```python
from build123d import *

# Parameters (mm, degrees)
SKETCH1_R           = 12.7
BOSS_EXTRUDE1_DEPTH = 58.7248
CHAMFER3_SIZE       = 6.35
CHAMFER3_SIZE2      = 23.698522628
CHAMFER4_SIZE       = 6.35
CHAMFER4_SIZE2      = 23.698522628
CUT_EXTRUDE1_DEPTH  = 58.7248
SKETCH3_R           = 1.5875
CUT_EXTRUDE2_DEPTH  = 62.409951433


with BuildPart() as part:
    # Sketch1 → Boss-Extrude1 (new body)
    with BuildSketch(Plane.XY):
        Circle(SKETCH1_R)
    extrude(amount=-BOSS_EXTRUDE1_DEPTH)

    # Chamfer3
    chamfer3_edges = [part.edges().sort_by_distance(p)[0] for p in [
        (-12.7, 0, -58.7248),
    ]]
    chamfer3_side = [part.faces().sort_by_distance(p)[0] for p in [
        (0, 0, -58.7248),
    ]]
    chamfer(chamfer3_edges, length=CHAMFER3_SIZE, length2=CHAMFER3_SIZE2, reference=chamfer3_side[0])

    # Chamfer4
    chamfer4_edges = [part.edges().sort_by_distance(p)[0] for p in [
        (-12.7, 0, 0),
    ]]
    chamfer4_side = [part.faces().sort_by_distance(p)[0] for p in [
        (0, 0, 0),
    ]]
    chamfer(chamfer4_edges, length=CHAMFER4_SIZE, length2=CHAMFER4_SIZE2, reference=chamfer4_side[0])

    # Sketch2 → Cut-Extrude1 (cut)
    with BuildSketch(Plane(origin=(0, 0, 0), x_dir=(1, 0, 0), z_dir=(0, 1, 0))):
        Polygon((-6.35, 0), (-12.7, 23.698522628), (-12.7, 35.026277372), (-6.35, 58.7248), (6.35, 58.7248), (12.7, 35.026277372), (12.7, 23.698522628), (6.35, 0), align=None)
    extrude(amount=-CUT_EXTRUDE1_DEPTH, mode=Mode.SUBTRACT)

    # Sketch3 → Cut-Extrude2 (cut, through all)
    with BuildSketch(Plane(origin=(0, 0, 0), x_dir=(1, 0, 0), z_dir=(0, 1, 0))):
        with Locations(Location((-10.16, 35.026277372, 0), (0, 0, 179.999999983))):
            Circle(SKETCH3_R)
        with Locations(Location((10.16, 35.026277372, 0), (0, 0, 90))):
            Circle(SKETCH3_R)
        with Locations((10.16, 23.698522628)):
            Circle(SKETCH3_R)
        with Locations(Location((-10.16, 23.698522628, 0), (0, 0, 90))):
            Circle(SKETCH3_R)
    extrude(amount=CUT_EXTRUDE2_DEPTH, mode=Mode.SUBTRACT)


solid = part.part
```
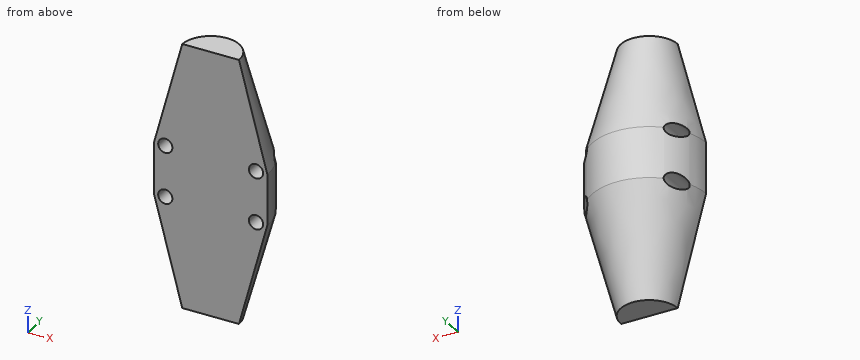
Here's how the part is built. I have some questions about the finished solid (model axes, mm). Coordinates: 2 decimals unless noted, no trailing zeros. Order: outer loops, then holes, each group sorted by start corner. A loop starts at its lowest first (then second) coordinate and runs counter-clockwise, first axis right, second up. Notation, with made-up numbers: M -29.75,-36.75 L 13.25,-36.75 A26 ccw 13.25,-3.75 Z; hole C 18,-3 d10. An arc over 180 degrees is marked long. Answer as a JSON object with one key per item and string values. Group by question number.
(1) Suppose I cut it at A-A, the plane x = 0. Please give me the cut outline in (y, z), then the cut area to 3 significant figures.
(2) Suppose I cut it at B-B, the plane y = 4. State how many separate pieces and enclosed holes the cut face has, then the cut area to 3 significant figures.
(3) For pin 1 (3 mm diameter, centred on x = -9, z = -27.5, fed in from -Y); pin 2 (2 mm diameter, centred on y = 11, z = -41.5, fed in from +X); pin 3 (1.5 mm diameter, centred on y = 8.5, z = -39.5, fed in from +X); pin 4 (3 mm diameter, centred on y = 2.5, z = -42.5, fed in from -X), each with a flat end and sliding along its axis, tell me the tip position at first contact or that it passes through.
(4) I need wall thicknesses on probe 1 along X at (y, z) = (1.5, -36); probe 2 along Y at (x, z) = (-4.25, -10); probe 3 along Y at (x, z) = (8.75, -31.5). Which ranges of each line are inside material? Lowest first, please.
(5) Suppose I cut it at D-D, the plane z = -54. Please give me the cut outline in (x, y), then the cut area to 3 significant figures.
Values found:
{
 "1": {"outline": "M 0,-58.72 L 6.35,-58.72 L 12.7,-35.03 L 12.7,-23.7 L 6.35,0 L 0,0 Z", "area": "595 mm^2"},
 "2": {"separate pieces": "1", "enclosed holes": "4", "area": "1,060 mm^2"},
 "3": {"pin 1": "stops at y = 0", "pin 2": "stops at x = 4.59", "pin 3": "stops at x = 8.55", "pin 4": "stops at x = -10.91"},
 "4": {"probe 1": "x = -12.35 to -11.41, -8.91 to 8.91, 11.41 to 12.35", "probe 2": "y = 0 to 7.97", "probe 3": "y = 0 to 9.2"},
 "5": {"outline": "M -7.62,0 L 7.62,0 A7.62 ccw Z", "area": "91.1 mm^2"}
}
